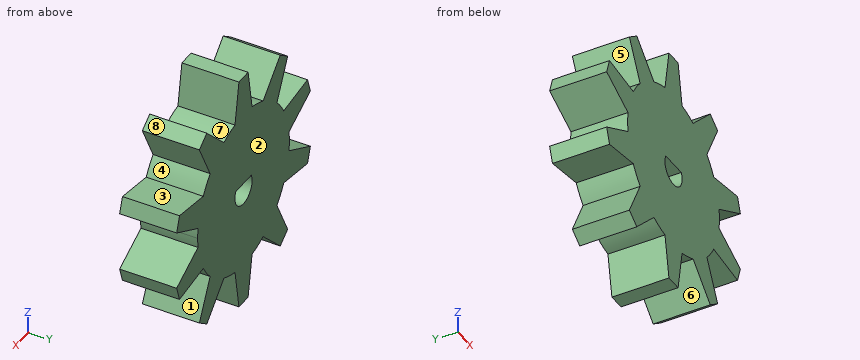
```python
from build123d import *

# Parameters (mm, degrees)
BOSS_EXTRUDE2_DEPTH = 7
CUT_EXTRUDE1_DEPTH  = 7


with BuildPart() as part:
    # Sketch1 → Boss-Extrude2 (new body)
    with BuildSketch(Plane(origin=(0, 0, 0), x_dir=(1, 0, 0), z_dir=(0, 1, 0))):
        with BuildLine():
            Line((-2, 9), (-1.862495894, 9.825024633))
            ThreePointArc((-1.862495894, 9.825024633), (-3.090169944, 9.510565163), (-4.268213752, 9.043359518))
            Line((-4.268213752, 9.043359518), (-3.672033282, 8.456723454))
            Line((-3.672033282, 8.456723454), (-6.908101259, 6.105582445))
            Line((-6.908101259, 6.105582445), (-7.281795413, 6.853864279))
            ThreePointArc((-7.281795413, 6.853864279), (-8.090169944, 5.877852523), (-8.768610817, 4.807438439))
            Line((-8.768610817, 4.807438439), (-7.941474658, 4.683265982))
            Line((-7.941474658, 4.683265982), (-9.177542635, 0.879039917))
            Line((-9.177542635, 0.879039917), (-9.919696584, 1.264760725))
            ThreePointArc((-9.919696584, 1.264760725), (-10, 0), (-9.919696584, -1.264760725))
            Line((-9.919696584, -1.264760725), (-9.177542635, -0.879039917))
            Line((-9.177542635, -0.879039917), (-7.941474658, -4.683265982))
            Line((-7.941474658, -4.683265982), (-8.768610817, -4.807438439))
            ThreePointArc((-8.768610817, -4.807438439), (-8.090169944, -5.877852523), (-7.281795413, -6.853864279))
            Line((-7.281795413, -6.853864279), (-6.908101259, -6.105582445))
            Line((-6.908101259, -6.105582445), (-3.672033282, -8.456723454))
            Line((-3.672033282, -8.456723454), (-4.268213752, -9.043359518))
            ThreePointArc((-4.268213752, -9.043359518), (-3.090169944, -9.510565163), (-1.862495894, -9.825024633))
            Line((-1.862495894, -9.825024633), (-2, -9))
            Line((-2, -9), (2, -9))
            Line((2, -9), (1.862495894, -9.825024633))
            ThreePointArc((1.862495894, -9.825024633), (3.090169944, -9.510565163), (4.268213752, -9.043359518))
            Line((4.268213752, -9.043359518), (3.672033282, -8.456723454))
            Line((3.672033282, -8.456723454), (6.908101259, -6.105582445))
            Line((6.908101259, -6.105582445), (7.281795413, -6.853864279))
            ThreePointArc((7.281795413, -6.853864279), (8.090169944, -5.877852523), (8.768610817, -4.807438439))
            Line((8.768610817, -4.807438439), (7.941474658, -4.683265982))
            Line((7.941474658, -4.683265982), (9.177542635, -0.879039917))
            Line((9.177542635, -0.879039917), (9.919696584, -1.264760725))
            ThreePointArc((9.919696584, -1.264760725), (9.979903953, -0.633653756), (10, 0))
            ThreePointArc((10, 0), (9.979903953, 0.633653756), (9.919696584, 1.264760725))
            Line((9.919696584, 1.264760725), (9.177542635, 0.879039917))
            Line((9.177542635, 0.879039917), (7.941474658, 4.683265982))
            Line((7.941474658, 4.683265982), (8.768610817, 4.807438439))
            ThreePointArc((8.768610817, 4.807438439), (8.090169944, 5.877852523), (7.281795413, 6.853864279))
            Line((7.281795413, 6.853864279), (6.908101259, 6.105582445))
            Line((6.908101259, 6.105582445), (3.672033282, 8.456723454))
            Line((3.672033282, 8.456723454), (4.268213752, 9.043359518))
            ThreePointArc((4.268213752, 9.043359518), (3.090169944, 9.510565163), (1.862495894, 9.825024633))
            Line((1.862495894, 9.825024633), (2, 9))
            Line((2, 9), (-2, 9))
        make_face()
        with BuildLine():
            ThreePointArc((-8.768610817, -4.807438439), (-9.510565163, -3.090169944), (-9.919696584, -1.264760725))
            Line((-9.919696584, -1.264760725), (-14.574864739, -3.684198399))
            Line((-14.574864739, -3.684198399), (-13.95683075, -5.586311432))
            Line((-13.95683075, -5.586311432), (-8.768610817, -4.807438439))
        make_face()
        with BuildLine():
            ThreePointArc((-4.268213752, -9.043359518), (-5.877852523, -8.090169944), (-7.281795413, -6.853864279))
            Line((-7.281795413, -6.853864279), (-9.625795779, -11.547469663))
            Line((-9.625795779, -11.547469663), (-8.00776179, -12.723040168))
            Line((-8.00776179, -12.723040168), (-4.268213752, -9.043359518))
        make_face()
        with BuildLine():
            ThreePointArc((1.862495894, -9.825024633), (0, -10), (-1.862495894, -9.825024633))
            Line((-1.862495894, -9.825024633), (-1, -15))
            Line((-1, -15), (1, -15))
            Line((1, -15), (1.862495894, -9.825024633))
        make_face()
        with BuildLine():
            Line((9.625795779, -11.547469663), (7.281795413, -6.853864279))
            ThreePointArc((7.281795413, -6.853864279), (5.877852523, -8.090169944), (4.268213752, -9.043359518))
            Line((4.268213752, -9.043359518), (8.00776179, -12.723040168))
            Line((8.00776179, -12.723040168), (9.625795779, -11.547469663))
        make_face()
        with BuildLine():
            Line((14.574864739, -3.684198399), (9.919696584, -1.264760725))
            ThreePointArc((9.919696584, -1.264760725), (9.510565163, -3.090169944), (8.768610817, -4.807438439))
            Line((8.768610817, -4.807438439), (13.95683075, -5.586311432))
            Line((13.95683075, -5.586311432), (14.574864739, -3.684198399))
        make_face()
        with BuildLine():
            Line((13.95683075, 5.586311432), (8.768610817, 4.807438439))
            ThreePointArc((8.768610817, 4.807438439), (9.510565163, 3.090169944), (9.919696584, 1.264760725))
            Line((9.919696584, 1.264760725), (14.574864739, 3.684198399))
            Line((14.574864739, 3.684198399), (13.95683075, 5.586311432))
        make_face()
        with BuildLine():
            Line((8.00776179, 12.723040168), (4.268213752, 9.043359518))
            ThreePointArc((4.268213752, 9.043359518), (5.877852523, 8.090169944), (7.281795413, 6.853864279))
            Line((7.281795413, 6.853864279), (9.625795779, 11.547469663))
            Line((9.625795779, 11.547469663), (8.00776179, 12.723040168))
        make_face()
        with BuildLine():
            Line((1, 15), (-1, 15))
            Line((-1, 15), (-1.862495894, 9.825024633))
            ThreePointArc((-1.862495894, 9.825024633), (0, 10), (1.862495894, 9.825024633))
            Line((1.862495894, 9.825024633), (1, 15))
        make_face()
        with BuildLine():
            ThreePointArc((-7.281795413, 6.853864279), (-5.877852523, 8.090169944), (-4.268213752, 9.043359518))
            Line((-4.268213752, 9.043359518), (-8.00776179, 12.723040168))
            Line((-8.00776179, 12.723040168), (-9.625795779, 11.547469663))
            Line((-9.625795779, 11.547469663), (-7.281795413, 6.853864279))
        make_face()
        with BuildLine():
            ThreePointArc((-9.919696584, 1.264760725), (-9.510565163, 3.090169944), (-8.768610817, 4.807438439))
            Line((-8.768610817, 4.807438439), (-13.95683075, 5.586311432))
            Line((-13.95683075, 5.586311432), (-14.574864739, 3.684198399))
            Line((-14.574864739, 3.684198399), (-9.919696584, 1.264760725))
        make_face()
        with BuildLine():
            Line((-7.941474658, 4.683265982), (-8.768610817, 4.807438439))
            ThreePointArc((-8.768610817, 4.807438439), (-9.510565163, 3.090169944), (-9.919696584, 1.264760725))
            Line((-9.919696584, 1.264760725), (-9.177542635, 0.879039917))
            Line((-9.177542635, 0.879039917), (-7.941474658, 4.683265982))
        make_face()
        with BuildLine():
            Line((-2, -9), (-1.862495894, -9.825024633))
            ThreePointArc((-1.862495894, -9.825024633), (0, -10), (1.862495894, -9.825024633))
            Line((1.862495894, -9.825024633), (2, -9))
            Line((2, -9), (-2, -9))
        make_face()
        with BuildLine():
            ThreePointArc((4.268213752, -9.043359518), (5.877852523, -8.090169944), (7.281795413, -6.853864279))
            Line((7.281795413, -6.853864279), (6.908101259, -6.105582445))
            Line((6.908101259, -6.105582445), (3.672033282, -8.456723454))
            Line((3.672033282, -8.456723454), (4.268213752, -9.043359518))
        make_face()
        with BuildLine():
            Line((-6.908101259, -6.105582445), (-7.281795413, -6.853864279))
            ThreePointArc((-7.281795413, -6.853864279), (-5.877852523, -8.090169944), (-4.268213752, -9.043359518))
            Line((-4.268213752, -9.043359518), (-3.672033282, -8.456723454))
            Line((-3.672033282, -8.456723454), (-6.908101259, -6.105582445))
        make_face()
        with BuildLine():
            Line((-9.177542635, -0.879039917), (-9.919696584, -1.264760725))
            ThreePointArc((-9.919696584, -1.264760725), (-9.510565163, -3.090169944), (-8.768610817, -4.807438439))
            Line((-8.768610817, -4.807438439), (-7.941474658, -4.683265982))
            Line((-7.941474658, -4.683265982), (-9.177542635, -0.879039917))
        make_face()
        with BuildLine():
            Line((-3.672033282, 8.456723454), (-4.268213752, 9.043359518))
            ThreePointArc((-4.268213752, 9.043359518), (-5.877852523, 8.090169944), (-7.281795413, 6.853864279))
            Line((-7.281795413, 6.853864279), (-6.908101259, 6.105582445))
            Line((-6.908101259, 6.105582445), (-3.672033282, 8.456723454))
        make_face()
        with BuildLine():
            ThreePointArc((1.862495894, 9.825024633), (0, 10), (-1.862495894, 9.825024633))
            Line((-1.862495894, 9.825024633), (-2, 9))
            Line((-2, 9), (2, 9))
            Line((2, 9), (1.862495894, 9.825024633))
        make_face()
        with BuildLine():
            ThreePointArc((7.281795413, 6.853864279), (5.877852523, 8.090169944), (4.268213752, 9.043359518))
            Line((4.268213752, 9.043359518), (3.672033282, 8.456723454))
            Line((3.672033282, 8.456723454), (6.908101259, 6.105582445))
            Line((6.908101259, 6.105582445), (7.281795413, 6.853864279))
        make_face()
        with BuildLine():
            ThreePointArc((9.919696584, 1.264760725), (9.510565163, 3.090169944), (8.768610817, 4.807438439))
            Line((8.768610817, 4.807438439), (7.941474658, 4.683265982))
            Line((7.941474658, 4.683265982), (9.177542635, 0.879039917))
            Line((9.177542635, 0.879039917), (9.919696584, 1.264760725))
        make_face()
        with BuildLine():
            ThreePointArc((8.768610817, -4.807438439), (9.510565163, -3.090169944), (9.919696584, -1.264760725))
            Line((9.919696584, -1.264760725), (9.177542635, -0.879039917))
            Line((9.177542635, -0.879039917), (7.941474658, -4.683265982))
            Line((7.941474658, -4.683265982), (8.768610817, -4.807438439))
        make_face()
    extrude(amount=BOSS_EXTRUDE2_DEPTH)

    # Sketch3 → Cut-Extrude1 (cut)
    with BuildSketch(Plane.XZ):
        with BuildLine():
            Line((-1.683745824, 0.825), (1.683745824, 0.825))
            ThreePointArc((1.683745824, 0.825), (0, -1.875), (-1.683745824, 0.825))
        make_face()
    extrude(amount=-CUT_EXTRUDE1_DEPTH, mode=Mode.SUBTRACT)


solid = part.part
```
Geometry check sheet. Reference: the model listing, model coordinates, mm. Face numbers are marked on the shaded views. A direction names the side the tool comes from. Coordinates: 2 decimals unless noted, no trailing zeros. Write each loop counter-clockwise with the first axis right and the second up, starting at its lowest first coordinate (ties: lowest second). Pieces come first, ordered by that corner, then holes. Notation, with made-up numbers: M 5.5,-9.5 L 39.5,-9.5 A11 cw 39.5,9.5 Z; hole C -20,-3 d10. An arc over 180 degrees is marked long. One line per item, written item: value. Start each with the question number.
(1) Sectioned sample at C-C, the plane z = 7.5. Enter the section's corners in (x, y), and give its area (3 significant figures).
(2) Scan lines: line 1 along X through (y, z) = (2.5, 12.5); line 2 along Z through (x, y) = (0, 5.25) (3 decimals); line 3 along X through (y, z) = (4.25, 12). Record each from-to range of solid material in increasing order. Write a range as [from, to].
(3) Sectioned sample at B-B, the plane x = -3. Enter the section's corners in (y, z).
(4) Release check for a two-part mould opening along X. For the marked faces 1, 2 and 3 record: released by +X, released by -X, zero draft, split by the parting line, or undercut.
(5) Tool access check on the marked faces 4, 5, 6, 7 and 8. Record the directions out of +Z, -Z, +X, -X, +Y, -Y that give a thin tool (end or side, any length) a straight path to the whole face; none if there is none.
(6) Sectioned sample at A-A, the plane x = 0. Enter the section's corners in (y, z) (3 decimals).
(7) Depth check by flat-ended pin: pin 1 (1 mm diameter, centred on x = -2.5, y = 2, fed in from +Z); pin 2 (1.5 mm diameter, centred on x = -11.5, y = 1.5, fed in from +Z); pin 3 (1.5 mm diameter, centred on x = 10, y = 2.5, fed in from +Z). Enter the tip coordinate at first touch or a pass-through.
Filled sheet:
1. outline: M -7.6,0 L 7.6,0 L 7.6,7 L -7.6,7 Z
1. area: 106 mm²
2. line 1: [-8.31, -7.78], [-1.42, 1.42], [7.78, 8.31]
2. line 2: [-15, -1.875], [0.825, 15]
2. line 3: [-9, -7.27], [-1.5, 1.5], [7.27, 9]
3. outline: M 0,-9.54 L 7,-9.54 L 7,9.54 L 0,9.54 Z
4. face 1: released by +X
4. face 2: zero draft
4. face 3: undercut
5. face 4: +Y, -Y
5. face 5: -X, +Y, -Y
5. face 6: -Z, +Y, -Y
5. face 7: +Z, +Y, -Y
5. face 8: +Z, +X, +Y, -Y
6. outline: M 0,-15 L 7,-15 L 7,-1.875 L 0,-1.875 Z; M 0,0.825 L 7,0.825 L 7,15 L 0,15 Z
7. pin 1: z = 9.8
7. pin 2: z = 5.33
7. pin 3: z = 11.82
